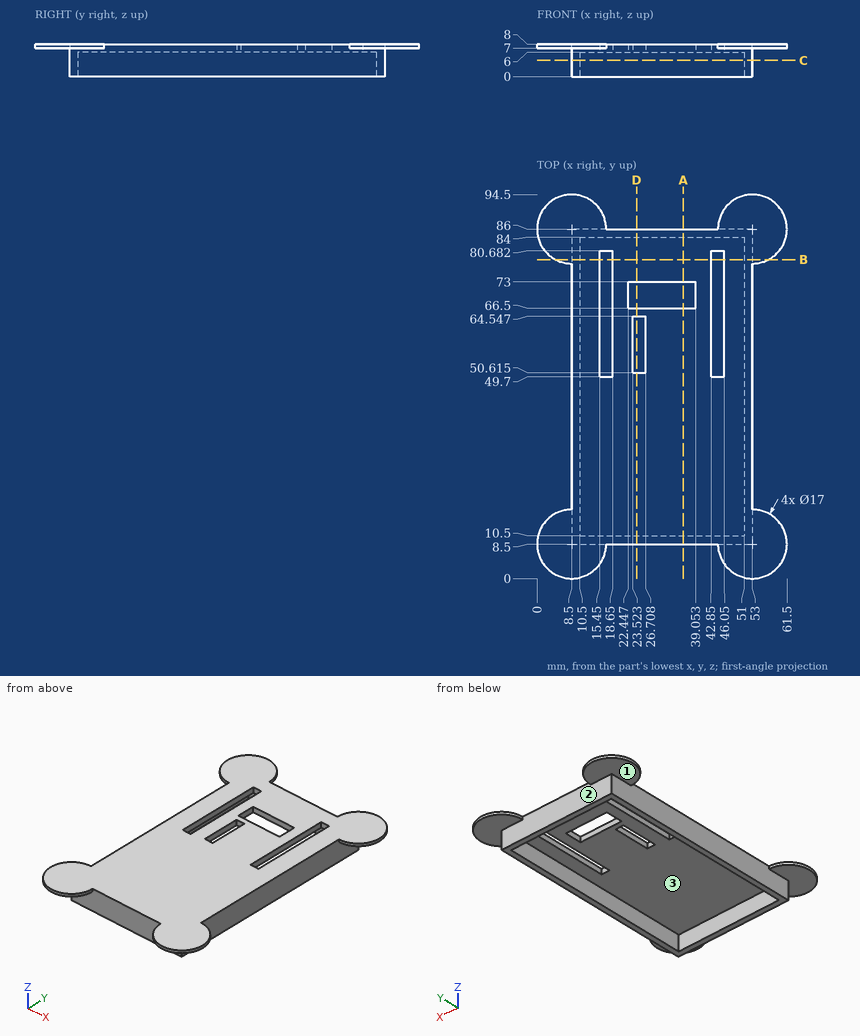
Can you work these out from the drawing? Everything is in mm from the part's minimum corner. Coordinates: 2 decimals unless noted, no trailing zeros. Loops run counter-clockwise (first coordinate to the right, second up) from the corner with the lowest first, then second, coordinate; pieces in that order, holes last. Notation, with made-up numbers: (-27.5, 42.5) - (-15.5, 42.5) arc R28 cw to (-15.5, 74.5) - close; hole circle Ø3 at (10, -27.75). An arc over 180 degrees is marked (long way). Put each result on its own line as item: value. Start each with the question number.
Item 1: Suppose I cut it at C-C (z = 4). Please give me the cut outline in (x, y).
Item 2: If I drill on line 1 along X through (y, z) = (54.5, 7.5); line 2 along X through (y, z) = (76.5, 7); line 3 along Y through (x, z) = (26, 7.5) (1 decimal), over which ranges is the centre line in solid material (lowest first)?
Item 3: Suppose I cut it at B-B (y = 78.5). Please give me the cut outline in (x, z), and give its area (3 significant figures).
Item 4: Suppose I cut it at D-D (x = 24.5). Please give me the cut outline in (y, z) (1 decimal).
Item 5: For pin 1 (5 mm diameter, centred on x = 56.5, y = 7, fed in from -Z); pin 2 (1.6 mm diameter, centred on x = 26, z = 7, fed in from +Y); pin 3 (1.6 mm diameter, centred on y = 69.5, z = 6.5, fed in from +X), each with a flat end and sliding along its axis, tell me the tip position at first contact or that it passes through.
Item 6: If we mould it in two halves opening along Y, with no side actions, what happens to the marked faces 1, 2 and 3? For each: +Y half, -Y half, draft (parallel to the pull), parting line (faces both ways), or undercut.
Item 7: Suppose I cut it at A-A (x = 36). Please give me the cut outline in (y, z).
Here are the results:
1. outline: (8.5, 8.5) - (53, 8.5) - (53, 86) - (8.5, 86) - close; hole (10.5, 10.5) - (51, 10.5) - (51, 84) - (10.5, 84) - close
2. line 1: 8.5 to 15.45, 18.65 to 23.52, 26.71 to 42.85, 46.05 to 53
2. line 2: 8.5 to 15.45, 18.65 to 42.85, 46.05 to 53
2. line 3: 8.5 to 50.6, 64.5 to 66.5, 73 to 86
3. outline: (4.5, 7) - (8.5, 7) - (8.5, 0) - (10.5, 0) - (10.5, 6) - (15.45, 6) - (15.45, 8) - (4.5, 8) - close; (18.65, 6) - (42.85, 6) - (42.85, 8) - (18.65, 8) - close; (46.05, 6) - (51, 6) - (51, 0) - (53, 0) - (53, 7) - (57, 7) - (57, 8) - (46.05, 8) - close
3. area: 108 mm²
4. outline: (8.5, 0) - (10.5, 0) - (10.5, 6) - (50.6, 6) - (50.6, 8) - (8.5, 8) - close; (64.5, 6) - (66.5, 6) - (66.5, 8) - (64.5, 8) - close; (73, 6) - (84, 6) - (84, 0) - (86, 0) - (86, 8) - (73, 8) - close
5. pin 1: z = 7
5. pin 2: y = 86
5. pin 3: x = 53
6. face 1: draft
6. face 2: +Y half
6. face 3: undercut
7. outline: (8.5, 0) - (10.5, 0) - (10.5, 6) - (66.5, 6) - (66.5, 8) - (8.5, 8) - close; (73, 6) - (84, 6) - (84, 0) - (86, 0) - (86, 8) - (73, 8) - close
